Autodesk Inventor part; units mm, degrees
ref_plane "YZ Plane" through (0, 0, 0) normal (1, 0, 0) x (0, 1, 0)
ref_plane "XZ Plane" through (0, 0, 0) normal (0, 1, 0) x (-1, 0, 0)
ref_plane "XY Plane" through (0, 0, 0) normal (0, 0, 1) x (1, 0, 0)
sketch "Sketch1" plane through (0, 0, 0) normal (0, 1, 0) x (-1, 0, 0)
  arc A0 (31.75, 0) -> (-31.75, 0) centre (0, 0) ccw
  line L0 (0, 0) -> (-31.75, 0) construction
  line L1 (0, 0) -> (31.75, 0) construction
  line L2 (31.75, 0) -> (-31.75, 0)
  dimension "d0" = 31.75
  dimension "d1" = 180
revolve "Revolution1" add sketch "Sketch1" angle 180 about axis through (-31.75, 0, 0) along (1, 0, 0)
sketch "Sketch2" plane through (0, 0, 0) normal (0, 1, 0) x (1, 0, 0)
  line L0 (0, 0) -> (0, 27.94)
  line L1 (0, 0) -> (0, 25.4)
  circle A0 centre (0, 0) radius 27.94
  circle A1 centre (0, 0) radius 25.4
  dimension "d3" = 27.94
  dimension "d4" = 25.4
extrude "Extrusion1" add sketch "Sketch2" along normal blind 3.175
sketch "Sketch3" plane through (0, 0, 0) normal (0, 1, 0) x (1, 0, 0)
  circle A0 centre (0, 0) radius 27.94
  circle A1 centre (0, 0) radius 31.75
extrude "Extrusion2" cut sketch "Sketch3" against normal blind 3.175
properties part number "bottom ball bottom"
Verification items for the finished model (mm, model axes). Coordinates: 2 decimals unless noted, no trailing zeros. Order: outer loops, then holes, each group sorted by start corner. A loop starts at its lowest first (then second) coordinate and runs counter-clockwise, first axis right, second up. Notation, with made-up numbers: M -33.5,83.5 L -5.5,83.5 A6 ccw -5.5,93.5 Z; hole C 3,26.5 d10. An arc over 180 degrees is marked long. One line per item, written item: value. Start each with the question number.
Item 1: Sectioned sample at C-C (y = 1). Enter the section's corners in (x, z), then the cut area to 3 significant figures.
Item 2: Scan lines: probe 1 along X at (y, z) = (1.65, 0); probe 2 along X at (y, z) = (-25.5, -6.5). Record each from-to range of solid material in increasing order.
Item 3: Gauge pin test, flat ends, axial feed: pin 1 (10 mm diameter, centred on y = -5.5, z = 22.5, fed in from -X); pin 2 (4 mm diameter, centred on x = 4.5, z = -20.5, fed in from +Y); pin 3 (6 mm diameter, centred on x = 4.5, y = -12, fed in from -Z); pin 4 (5 mm diameter, centred on x = 1, y = -3, fed in from +Z). Record the tip position at first contact, or that the pin passes through.
Item 4: Sectioned sample at D-D (y = -19). Enter the section's corners in (x, z).
Item 5: Mould release check, pull along X, two halves, no side actions. Record for faces 1 (the flat face through (6, 3.175, 25)), 2 (the cylindrical face through (-5.506, 1.565, -24.796)), 3 (the flat face through (0, 0, 0)): released by +X, released by -X, zero draft, split by the parting line, or undercut.
Item 6: Sectioned sample at A-A (x = 0). Enter the section's corners in (y, z) (3 decimals).
Item 7: Sectioned sample at B-B (z = 17). Enter the section's corners in (x, y) (3 decimals), then the cut area to 3 significant figures.
Conclusion:
1. outline: C 0,0 d55.88; hole C 0,0 d50.8
1. area: 426 mm^2
2. probe 1: x = -27.94 to -25.4, 25.4 to 27.94
2. probe 2: x = -17.76 to 17.76
3. pin 1: stops at x = -26.04
3. pin 2: stops at y = 0
3. pin 3: stops at z = -30.19
3. pin 4: stops at z = 31.59
4. outline: C 0,0 d50.87
5. face 1: zero draft
5. face 2: undercut
5. face 3: undercut
6. outline: M -3.175,-31.591 L -3.175,-27.94 L 3.175,-27.94 L 3.175,-25.4 L 0,-25.4 L 0,25.4 L 3.175,25.4 L 3.175,27.94 L -3.175,27.94 L -3.175,31.591 A31.75 ccw Z
7. outline: M -26.627,-3.175 A26.815 ccw 26.627,-3.175 L 22.173,-3.175 L 22.173,3.175 L 18.872,3.175 L 18.872,0 L -18.872,0 L -18.872,3.175 L -22.173,3.175 L -22.173,-3.175 Z
7. area: 1,120 mm^2
